Could you check a few things on this model? Use its own coordinates, in mm. Face numbers are marked on the shaded views. A direction names the side the tool comes from. Round coordinates to 2 decimals unless told otherwise and drop trailing zeros. Write each loop counter-clockwise with the first axis right and the second up, starting at its lowest first coordinate (ties: lowest second). Pieces come first, ordered by that corner, then holes. Notation, with made-up numbers: (24, 20.5) -> (79, 20.5) arc R26 cw to (79, 47.5) -> close; hole circle Ø1 at (-5, 75.5). An arc over 180 degrees is marked (long way). One line per question, with ' | ' between items. Start each with the question number.
1. Imagine slicing it at B-B, the plane y = 6.5. List the corners of the cut face in (x, z) for me.
2. Thinking about a two-plate mould opening in X: for the marked faces 3, 4, 5 and 6, which applies, released by +X, released by -X, zero draft, split by the parting line, or undercut?
3. If I drill on line 1 along Y through (x, z) = (43.5, 50.5); line 2 along X through (y, z) = (-1, 43); line 3 along Z through (x, y) = (50.5, -7), over which ranges is the centre line in solid material (lowest first)? Write a range as [from, to].
4. Imagine slicing it at A-A, the plane x = 8. List the corners of the cut face in (y, z) for me.
5. For the marked faces 1 and 2, which set-ups out of +Z, -Z, +X, -X, +Y, -Y let a thin tool reach every point of the face, with its end or its side?
6. For pin 1 Ø4 at (x, y) = (15, 6.5) entering from +Z; pin 2 Ø23 at (x, z) = (34.34, 25) entering from -Y, each with a flat end and sliding along its axis, tell me the tip position at first contact or that it passes through.
7. Imagine slicing it at D-D, the plane x = 63.5. List the corners of the cut face in (y, z) for me, and give its area (3 significant figures).
8. Imagine slicing it at C-C, the plane z = 25. List the corners of the cut face in (x, y) for me, and give its area (3 significant figures).
from build123d import *

# Parameters (mm, degrees)
F0_W     = 68.672989
F0_H     = 50
F0_R     = 10
F1_DEPTH = 15
F2_R     = 5.609518
F3_DEPTH = 93.9


with BuildPart() as f1:
    # F0 (on Front) → F1 (new body, symmetric)
    with BuildSketch(Plane.XZ):
        with Locations((34.336495, 25)):
            Rectangle(F0_W, F0_H)
        Polygon((10.629317, 48.182614), (14.130936, 42.374947), (9.689576, 37.250041), (3.443045, 39.890342), (4.023837, 46.647044), align=None, mode=Mode.SUBTRACT)
        with Locations((34.336495, 25)):
            Circle(F0_R, mode=Mode.SUBTRACT)
    extrude(amount=F1_DEPTH, both=True)

    # F2 (on face) → F3 (join)
    with BuildSketch(Plane(origin=(0, 0, 0), x_dir=(1, 0, 0), z_dir=(0, 0, -1))):
        with Locations((43.091845, 5.679999)):
            Circle(F2_R)
    extrude(amount=-F3_DEPTH)


solid = f1.part
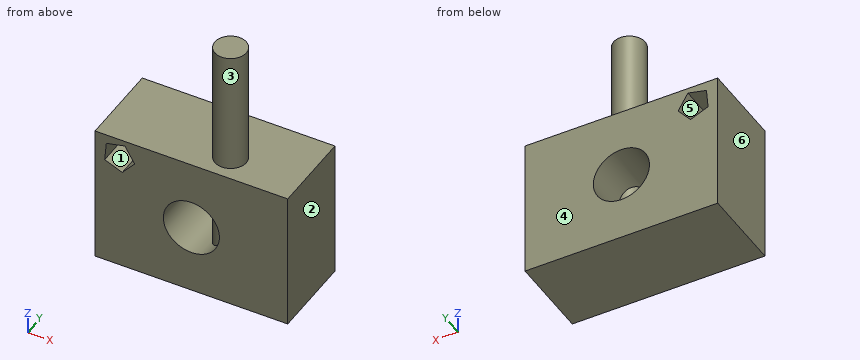
Geometry results:
1) outline: (0, 0) -> (68.67, 0) -> (68.67, 50) -> (0, 50) -> close; hole (3.44, 39.89) -> (9.69, 37.25) -> (14.13, 42.37) -> (10.63, 48.18) -> (4.02, 46.65) -> close; hole circle Ø20 at (34.34, 25)
2) face 3: split by the parting line | face 4: zero draft | face 5: undercut | face 6: released by -X
3) line 1: y = [-11.27, -0.09] | line 2: x = [0, 3.71], [13.75, 68.67] | line 3: z = [0, 50]
4) outline: (-15, 0) -> (15, 0) -> (15, 37.96) -> (-15, 37.96) -> close; (-15, 47.57) -> (15, 47.57) -> (15, 50) -> (-15, 50) -> close
5) face 1: +Y, -Y | face 2: +Z, -Z, +X, +Y, -Y
6) pin 1: stops at z = 50 | pin 2: stops at y = -15
7) outline: (-15, 0) -> (15, 0) -> (15, 50) -> (-15, 50) -> close | area: 1,500 mm2
8) outline: (0, -15) -> (24.34, -15) -> (24.34, 15) -> (0, 15) -> close; (44.34, -15) -> (68.67, -15) -> (68.67, 15) -> (44.34, 15) -> (44.34, -0.21) arc R5.61 ccw (long way) to (44.34, -11.15) -> close | area: 1,520 mm2
